Source: CAD feature listing. Evaluate the final solid. Frame: model axes, mm. Round coordinates to 2 decimals unless told otherwise and drop trailing zeros. Order: outer loops, then holes, each group sorted by start corner. A loop starts at its lowest first (then second) coordinate and runs counter-clockwise, first axis right, second up. Notation, with made-up numbers: (20.5, 85) - (48.5, 85) arc R5 ccw to (48.5, 90) - close; hole circle Ø1 at (32.5, -9). An arc over 180 degrees is marked (long way). Use one line per item in the form item = value. Start each with the question number.
Q1. Cut plane B-B, the plane z = -171. Return the cut outline in (x, y).
Q2. Ray query, line 1 (X direction, y = 5.25, z = -78); line 2 (Z direction, x = 201.75, y = 10); line 3 (Z direction, x = 102, y = 17.5). Return the intervals inside material, ascending. Write a range as [from, to].
Q3. Cut plane A-A, the plane z = -40. Return the cut outline in (x, y).
Q4. Pin query (flat end, axial travel): pin 1 Ø14.5 at (x, z) = (40, -255) entering from -Y. Return the tip coordinate at first contact, or that it passes through.
from build123d import *

# Parameters (mm, degrees)
FILLET1_OUTLINE_R     = 8
FILLET1_OUTLINE_R_2   = 7
FILLET1_OUTLINE_R_3   = 1.65
FILLET1_DEPTH         = 20
FILLET1_START         = 11
FILLET1_2_OUTLINE_R   = 7
FILLET1_2_OUTLINE_R_2 = 3
FILLET1_2_OUTLINE_R_3 = 1.65
FILLET1_2_DEPTH       = 9
FILLET1_START_2       = 10
FILLET1_3_OUTLINE_R   = 1.65
FILLET1_3_DEPTH       = 1
FILLET1_START_3       = -1
FILLET1_4_OUTLINE_R   = 2.5
FILLET1_4_DEPTH       = 289
CUT_EXTRUDE1_DEPTH    = 42
FILLET2_R             = 10
SKETCH2_W             = 42.909643268
SKETCH2_H             = 22.925607662
SKETCH2_W_2           = 43.116379367
SKETCH2_H_2           = 35.117017069
CUT_EXTRUDE2_DEPTH    = 42
FILLET3_R             = 5


with BuildPart() as part:
    # Fillet1: read off the stored shape, not the designer's step
    # Fillet1 outline → Fillet1 (new body)
    with BuildSketch(Plane(origin=(0, 0, 0), x_dir=(1, 0, 0), z_dir=(0, 1, 0))):
        Polygon((0, 280), (0, 10), (10, 0), (277, 0), (287, 10), (287, 280), (277, 290), (10, 290), align=None)
        with Locations((40, 40)):
            Circle(FILLET1_OUTLINE_R, mode=Mode.SUBTRACT)
        with Locations((143.495955763, 90)):
            Circle(FILLET1_OUTLINE_R_2, mode=Mode.SUBTRACT)
        with Locations((143.495955763, 124)):
            Circle(FILLET1_OUTLINE_R_2, mode=Mode.SUBTRACT)
        with Locations((247, 40)):
            Circle(FILLET1_OUTLINE_R, mode=Mode.SUBTRACT)
        with Locations((40, 255)):
            Circle(FILLET1_OUTLINE_R, mode=Mode.SUBTRACT)
        with Locations((133.495955763, 219.5)):
            Circle(FILLET1_OUTLINE_R_3, mode=Mode.SUBTRACT)
        with BuildLine():
            Line((237, 110), (222, 110))
            ThreePointArc((222, 110), (219.878679656, 109.121320344), (219, 107))
            Line((219, 107), (219, 73))
            ThreePointArc((219, 73), (218.121320344, 70.878679656), (216, 70))
            Line((216, 70), (214, 70))
            ThreePointArc((214, 70), (211.878679656, 70.878679656), (211, 73))
            Line((211, 73), (211, 107))
            ThreePointArc((211, 107), (210.121320344, 109.121320344), (208, 110))
            Line((208, 110), (196, 110))
            ThreePointArc((196, 110), (193.878679656, 109.121320344), (193, 107))
            Line((193, 107), (193, 73))
            ThreePointArc((193, 73), (192.121320344, 70.878679656), (190, 70))
            Line((190, 70), (178, 70))
            ThreePointArc((178, 70), (175.878679656, 70.878679656), (175, 73))
            Line((175, 73), (175, 137))
            ThreePointArc((175, 137), (174.121320344, 139.121320344), (172, 140))
            Line((172, 140), (116, 140))
            ThreePointArc((116, 140), (113.878679656, 139.121320344), (113, 137))
            Line((113, 137), (113, 73))
            ThreePointArc((113, 73), (112.121320344, 70.878679656), (110, 70))
            Line((110, 70), (98, 70))
            ThreePointArc((98, 70), (95.878679656, 70.878679656), (95, 73))
            Line((95, 73), (95, 107))
            ThreePointArc((95, 107), (94.121320344, 109.121320344), (92, 110))
            Line((92, 110), (80, 110))
            ThreePointArc((80, 110), (77.878679656, 109.121320344), (77, 107))
            Line((77, 107), (77, 73))
            ThreePointArc((77, 73), (76.121320344, 70.878679656), (74, 70))
            Line((74, 70), (72, 70))
            ThreePointArc((72, 70), (69.878679656, 70.878679656), (69, 73))
            Line((69, 73), (69, 107))
            ThreePointArc((69, 107), (68.121320344, 109.121320344), (66, 110))
            Line((66, 110), (50, 110))
            ThreePointArc((50, 110), (42.928932188, 112.928932188), (40, 120))
            Line((40, 120), (40, 190))
            ThreePointArc((40, 190), (45.857864376, 204.142135624), (60, 210))
            Line((60, 210), (61, 210))
            ThreePointArc((61, 210), (63.121320344, 210.878679656), (64, 213))
            Line((64, 213), (64, 239))
            ThreePointArc((64, 239), (64.878679656, 241.121320344), (67, 242))
            Line((67, 242), (69, 242))
            ThreePointArc((69, 242), (71.121320344, 241.121320344), (72, 239))
            Line((72, 239), (72, 213))
            ThreePointArc((72, 213), (72.878679656, 210.878679656), (75, 210))
            Line((75, 210), (109, 210))
            ThreePointArc((109, 210), (111.121320344, 210.878679656), (112, 213))
            Line((112, 213), (112, 239))
            ThreePointArc((112, 239), (112.878679656, 241.121320344), (115, 242))
            Line((115, 242), (117, 242))
            ThreePointArc((117, 242), (119.121320344, 241.121320344), (120, 239))
            Line((120, 239), (120, 213))
            ThreePointArc((120, 213), (120.878679656, 210.878679656), (123, 210))
            Line((123, 210), (165, 210))
            ThreePointArc((165, 210), (167.121320344, 210.878679656), (168, 213))
            Line((168, 213), (168, 239))
            ThreePointArc((168, 239), (168.878679656, 241.121320344), (171, 242))
            Line((171, 242), (173, 242))
            ThreePointArc((173, 242), (175.121320344, 241.121320344), (176, 239))
            Line((176, 239), (176, 213))
            ThreePointArc((176, 213), (176.878679656, 210.878679656), (179, 210))
            Line((179, 210), (213, 210))
            ThreePointArc((213, 210), (215.121320344, 210.878679656), (216, 213))
            Line((216, 213), (216, 239))
            ThreePointArc((216, 239), (216.878679656, 241.121320344), (219, 242))
            Line((219, 242), (221, 242))
            ThreePointArc((221, 242), (223.121320344, 241.121320344), (224, 239))
            Line((224, 239), (224, 213))
            ThreePointArc((224, 213), (224.878679656, 210.878679656), (227, 210))
            ThreePointArc((227, 210), (241.142135624, 204.142135624), (247, 190))
            Line((247, 190), (247, 120))
            ThreePointArc((247, 120), (244.071067812, 112.928932188), (237, 110))
        make_face(mode=Mode.SUBTRACT)
        with Locations((153.495955763, 219.5)):
            Circle(FILLET1_OUTLINE_R_3, mode=Mode.SUBTRACT)
        with Locations((247, 255)):
            Circle(FILLET1_OUTLINE_R, mode=Mode.SUBTRACT)
    extrude(amount=FILLET1_DEPTH)

    # Fillet1 2 outline → Fillet1 2 (add)
    # profile 1 of 4: a face of its own
    with BuildSketch(Plane(origin=(0, 0, 0), x_dir=(1, 0, 0), z_dir=(0, 1, 0)).offset(FILLET1_START)):
        with Locations((143.495955763, 90)):
            Circle(FILLET1_2_OUTLINE_R)
        with Locations((143.495955763, 90)):
            Circle(FILLET1_2_OUTLINE_R_2, mode=Mode.SUBTRACT)
    # profile 2 of 4: a face of its own
    with BuildSketch(Plane(origin=(0, 0, 0), x_dir=(1, 0, 0), z_dir=(0, 1, 0)).offset(FILLET1_START)):
        with Locations((143.495955763, 124)):
            Circle(FILLET1_2_OUTLINE_R)
        with Locations((143.495955763, 124)):
            Circle(FILLET1_2_OUTLINE_R_2, mode=Mode.SUBTRACT)
    # profile 3 of 4: a face of its own
    with BuildSketch(Plane(origin=(0, 0, 0), x_dir=(1, 0, 0), z_dir=(0, 1, 0)).offset(FILLET1_START)):
        with Locations((153.495955763, 219.5)):
            Circle(FILLET1_2_OUTLINE_R_3)
    # profile 4 of 4: a face of its own
    with BuildSketch(Plane(origin=(0, 0, 0), x_dir=(1, 0, 0), z_dir=(0, 1, 0)).offset(FILLET1_START)):
        with Locations((133.495955763, 219.5)):
            Circle(FILLET1_2_OUTLINE_R_3)
    extrude(amount=FILLET1_2_DEPTH)

    # Fillet1 3 outline → Fillet1 3 (add)
    with BuildSketch(Plane(origin=(0, 0, 0), x_dir=(1, 0, 0), z_dir=(0, 1, 0)).offset(FILLET1_START_2)):
        with Locations((153.495955763, 219.5)):
            Circle(FILLET1_3_OUTLINE_R)
        with Locations((133.495955763, 219.5)):
            Circle(FILLET1_3_OUTLINE_R)
    extrude(amount=FILLET1_3_DEPTH)

    # Fillet1 4 outline → Fillet1 4 (cut)
    with BuildSketch(Plane.YZ.offset(FILLET1_START_3)):
        with Locations((10, -77.99)):
            Circle(FILLET1_4_OUTLINE_R)
        with Locations((10, -229.99)):
            Circle(FILLET1_4_OUTLINE_R)
    extrude(amount=FILLET1_4_DEPTH, mode=Mode.SUBTRACT)

    # Sketch1 → Cut-Extrude1 (cut)
    with BuildSketch(Plane(origin=(0, 20, 0), x_dir=(1, 0, 0), z_dir=(0, 1, 0))):
        Polygon((113, 115), (126, 140), (126, 142.938588866), (102.686400204, 142.938588866), (102.686400204, 115), align=None)
        Polygon((175, 115), (162, 140), (162, 142.938588866), (181.775389982, 142.938588866), (181.775389982, 115), align=None)
    extrude(amount=-CUT_EXTRUDE1_DEPTH, mode=Mode.SUBTRACT)

    # Fillet2
    fillet2_edges = [part.edges().sort_by_distance(p)[0] for p in [
        (113, 10, -115),
        (175, 10, -115),
        (126, 10, -140),
        (162, 10, -140),
    ]]
    fillet(fillet2_edges, radius=FILLET2_R)

    # Sketch2 → Cut-Extrude2 (cut)
    with BuildSketch(Plane(origin=(0, 20, 0), x_dir=(1, 0, 0), z_dir=(0, 1, 0))):
        with Locations((93.454821634, 208.537196169)):
            Rectangle(SKETCH2_W, SKETCH2_H)
        with Locations((197.558189684, 203.14602613)):
            Rectangle(SKETCH2_W_2, SKETCH2_H_2)
    extrude(amount=-CUT_EXTRUDE2_DEPTH, mode=Mode.SUBTRACT)

    # Fillet3
    fillet3_edges = [part.edges().sort_by_distance(p)[0] for p in [
        (112, 10, -220),
        (72, 10, -220),
        (176, 10, -220.704534665),
        (216, 10, -220.704534665),
    ]]
    fillet(fillet3_edges, radius=FILLET3_R)


solid = part.part
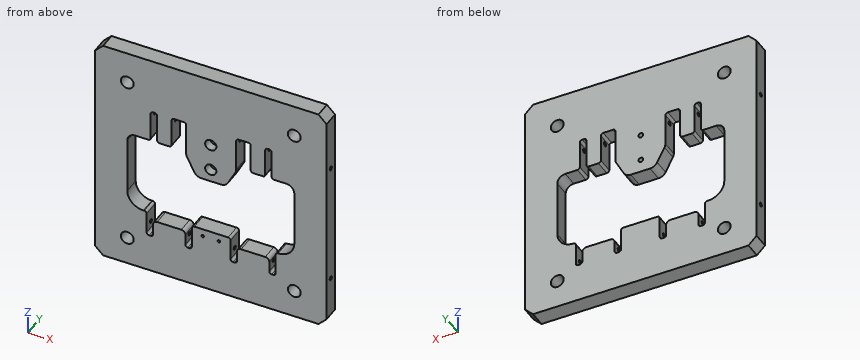
Completed:
q1.outline = (0, 0) - (40, 0) - (40, 20) - (0, 20) - close; (247, 0) - (287, 0) - (287, 20) - (247, 20) - close
q2.line_1 = [0, 69], [77, 95], [113, 175], [193, 211], [219, 287]
q2.line_2 = [-290, -232.49], [-227.49, -220.7], [-110, -80.49], [-75.49, 0]
q2.line_3 = [-290, -220], [-70, 0]
q3.outline = (0, 0) - (32, 0) - (32, 20) - (0, 20) - close; (48, 0) - (239, 0) - (239, 20) - (48, 20) - close; (255, 0) - (287, 0) - (287, 20) - (255, 20) - close
q4.pin_1 = through
